Geometry check sheet. Reference: the model listing, model coordinates, mm. Face numbers are marked on the shaded views. A direction names the side the tool comes from. Coordinates: 2 decimals unless noted, no trailing zeros. Write each loop counter-clockwise with the first axis right and the second up, starting at its lowest first coordinate (ties: lowest second). Pieces come first, ordered by that corner, then holes. Notation, with made-up numbers: (24, -4) -> (48, -4) arc R21 cw to (48, 34) -> close; hole circle Ø3 at (10, 76). An arc over 180 degrees is marked (long way). Use a Markdown table: item, result.
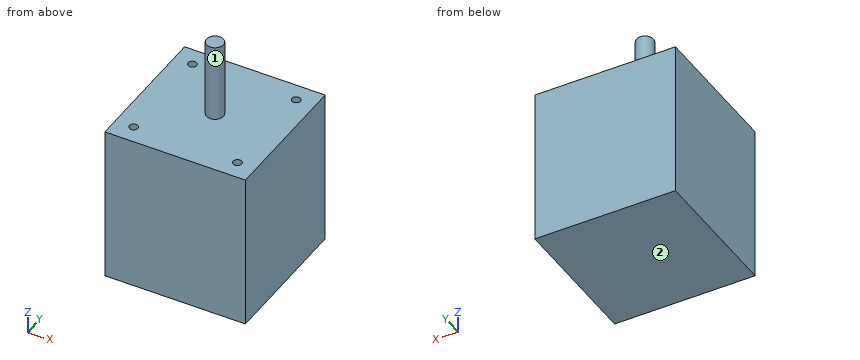
```python
from build123d import *

# Parameters (mm, degrees)
SKETCH1_W           = 42.0116
SKETCH1_H           = 42.01
BOSS_EXTRUDE1_DEPTH = 23.495
SKETCH2_R           = 2.54
BOSS_EXTRUDE2_DEPTH = 23.368
SKETCH3_R           = 1.27
CUT_EXTRUDE1_DEPTH  = 5.588


with BuildPart() as part:
    # Sketch1 → Boss-Extrude1 (new, symmetric)
    with BuildSketch(Plane.XY):
        Rectangle(SKETCH1_W, SKETCH1_H)
    extrude(amount=BOSS_EXTRUDE1_DEPTH, both=True)

    # Sketch2 → Boss-Extrude2 (add)
    with BuildSketch(Plane.XY.offset(23.495)):
        Circle(SKETCH2_R)
    extrude(amount=BOSS_EXTRUDE2_DEPTH)

    # Sketch3 → Cut-Extrude1 (cut)
    with BuildSketch(Plane.XY.offset(23.495)):
        with Locations((15.4686, -15.4678)):
            Circle(SKETCH3_R)
        with Locations((-15.5448, 15.5186)):
            Circle(SKETCH3_R)
        with Locations((15.4686, 15.5186)):
            Circle(SKETCH3_R)
        with Locations((-15.5448, -15.4678)):
            Circle(SKETCH3_R)
    extrude(amount=-CUT_EXTRUDE1_DEPTH, mode=Mode.SUBTRACT)


solid = part.part
```
Item 1: Section check D-D on x = -6.5. Record the boundary of the cut face in (y, z) (3 decimals), then the cut area to 3 significant figures.
Answer block:
| item | result |
|---|---|
| outline | (-21.005, -23.495) -> (21.005, -23.495) -> (21.005, 23.495) -> (-21.005, 23.495) -> close |
| area | 1,970 mm^2 |
Item 2: Thickness scan on L1, parallel to Z at x = -11.5, y = -0.5 (3 decimals). Record the ranges inside material, lowest first. Write a range as [from, to].
Answer block:
| item | result |
|---|---|
| L1 | z = [-23.495, 23.495] |
Item 3: Section check C-C on y = 12. Record the boundary of the cut face in (x, z) (3 decimals), then the cut area to 3 significant figures.
Answer block:
| item | result |
|---|---|
| outline | (-21.006, -23.495) -> (21.006, -23.495) -> (21.006, 23.495) -> (-21.006, 23.495) -> close |
| area | 1,970 mm^2 |
Item 4: Section check B-B on x = 0. Record the boundary of the cut face in (y, z) (3 decimals), then the cut area to 3 significant figures.
Answer block:
| item | result |
|---|---|
| outline | (-21.005, -23.495) -> (21.005, -23.495) -> (21.005, 23.495) -> (2.54, 23.495) -> (2.54, 46.863) -> (-2.54, 46.863) -> (-2.54, 23.495) -> (-21.005, 23.495) -> close |
| area | 2,090 mm^2 |
Item 5: Depth check by flat-ended pin: P1, Ø12.5, axis at x = -2, y = 6, coming from the +Z side; P2, Ø2, axis at x = -15, y = 16, coming from the +Z side (3 decimals); P3, Ø1.5, axis at x = -15.54, y = -15.47, coming from the +Z side; P4, Ø1.5, axis at y = 3, z = 35, coming from the -X side. Enter the tip coordinate at first touch or a pass-through.
Answer block:
| item | result |
|---|---|
| P1 | stops at z = 46.86 |
| P2 | stops at z = 23.495 |
| P3 | stops at z = 17.91 |
| P4 | stops at x = -1.18 |
Item 6: Tool access check on the marked faces 1 and 2. Record the directions out of +Z, -Z, +X, -X, +Y, -Y that give a thin tool (end or side, any length) a straight path to the whole face; none if there is none.
Answer block:
| item | result |
|---|---|
| face 1 | +Z |
| face 2 | -Z, +X, -X, +Y, -Y |
Item 7: Section check A-A on y = 0. Record the boundary of the cut face in (x, z) (3 decimals).
Answer block:
| item | result |
|---|---|
| outline | (-21.006, -23.495) -> (21.006, -23.495) -> (21.006, 23.495) -> (2.54, 23.495) -> (2.54, 46.863) -> (-2.54, 46.863) -> (-2.54, 23.495) -> (-21.006, 23.495) -> close |
